```python
from build123d import *

# Parameters (mm, degrees)
SKETCH_W           = 49
SKETCH_H           = 20
PAD_DEPTH          = 2
SKETCH001_W        = 10
SKETCH001_H        = 10
PAD001_DEPTH       = 5
SKETCH002_W        = 13.5
SKETCH002_H        = 10
POCKET_DEPTH       = 5
SKETCH003_W        = 3
SKETCH003_H        = 20
PAD002_DEPTH       = 10
SKETCH004_W        = 1
SKETCH004_H        = 2
PAD003_DEPTH       = 2
PAD003_FACE1_W     = 20
PAD003_FACE1_H     = 2
PAD004_DEPTH       = 2
SKETCH005_W        = 3
SKETCH005_H        = 20
PAD005_DEPTH       = 10
SKETCH006_W        = 1
SKETCH006_H        = 20
PAD006_DEPTH       = 2
PAD006_FACE9_W     = 10
PAD006_FACE9_H     = 2
POCKET001_DEPTH    = 5
SKETCH007_W        = 10
SKETCH007_H        = 2
POCKET002_DEPTH    = 5
POCKET002_FACE22_W = 20
POCKET002_FACE22_H = 1
PAD007_DEPTH       = 5
PAD007_FACE13_W    = 2
PAD007_FACE13_H    = 1
PAD008_DEPTH       = 5
PAD008_FACE22_W    = 2
PAD008_FACE22_H    = 1
PAD009_DEPTH       = 5
PAD009_FACE26_W    = 10
PAD009_FACE26_H    = 10
PAD010_DEPTH       = 15
SKETCH009_W        = 10
SKETCH009_H        = 2
PAD011_DEPTH       = 5
PAD011_FACE29_W    = 10
PAD011_FACE29_H    = 10
PAD012_DEPTH       = 3
SKETCH010_W        = 8
SKETCH010_H        = 2
POCKET003_DEPTH    = 15.001
CHAMFER_SIZE       = 1
CHAMFER_FACE27_W   = 10
CHAMFER_FACE27_H   = 2
PAD013_DEPTH       = 20


with BuildPart() as part:
    # Sketch → Pad (new body)
    with BuildSketch(Plane.XY):
        with Locations((24.5, 10)):
            Rectangle(SKETCH_W, SKETCH_H)
    extrude(amount=PAD_DEPTH)

    # Sketch001 (on Face6 of Pad) → Pad001 (join)
    with BuildSketch(Plane.XY.offset(2)):
        with Locations((24.5, 10)):
            Rectangle(SKETCH001_W, SKETCH001_H)
    extrude(amount=-PAD001_DEPTH)

    # Sketch002 (on Face4 of Pad001) → Pocket (cut)
    with BuildSketch(Plane(origin=(0, 0, 0), x_dir=(1, 0, 0), z_dir=(0, 0, -1))):
        with Locations((39.25, -10)):
            Rectangle(SKETCH002_W, SKETCH002_H)
        with Locations((9.75, -10)):
            Rectangle(SKETCH002_W, SKETCH002_H)
    extrude(amount=-POCKET_DEPTH, mode=Mode.SUBTRACT)

    # Sketch003 (on Face5 of Pocket) → Pad002 (join)
    with BuildSketch(Plane.XY.offset(2)):
        with Locations((47.5, 10)):
            Rectangle(SKETCH003_W, SKETCH003_H)
    extrude(amount=PAD002_DEPTH)

    # Sketch004 (on Face17 of Pad002) → Pad003 (join)
    with BuildSketch(Plane.XY.offset(12)):
        with Locations((48.5, 19)):
            Rectangle(SKETCH004_W, SKETCH004_H)
        with Locations((48.5, 1)):
            Rectangle(SKETCH004_W, SKETCH004_H)
    extrude(amount=PAD003_DEPTH)

    # Pad003 Face1 → Pad004 (add)
    with BuildSketch(Plane(origin=(0, 10, 1), x_dir=(0, 1, 0), z_dir=(-1, 0, 0))):
        Rectangle(PAD003_FACE1_W, PAD003_FACE1_H)
    extrude(amount=PAD004_DEPTH)

    # Sketch005 (on Face26 of Pad004) → Pad005 (join)
    with BuildSketch(Plane.XY.offset(2)):
        with Locations((-0.5, 10)):
            Rectangle(SKETCH005_W, SKETCH005_H)
    extrude(amount=PAD005_DEPTH)

    # Sketch006 (on Face22 of Pad005) → Pad006 (join)
    with BuildSketch(Plane.XY.offset(12)):
        with Locations((-1.5, 10)):
            Rectangle(SKETCH006_W, SKETCH006_H)
    extrude(amount=PAD006_DEPTH)

    # Pad006 Face9 → Pocket001 (cut)
    with BuildSketch(Plane(origin=(3, 10, 1), x_dir=(0, -1, 0), z_dir=(1, 0, 0))):
        Rectangle(PAD006_FACE9_W, PAD006_FACE9_H)
    extrude(amount=-POCKET001_DEPTH, mode=Mode.SUBTRACT)

    # Sketch007 (on Face8 of Pocket001) → Pocket002 (cut)
    with BuildSketch(Plane(origin=(46, 0, 0), x_dir=(0, -1, 0), z_dir=(-1, 0, 0))):
        with Locations((-10, 1)):
            Rectangle(SKETCH007_W, SKETCH007_H)
    extrude(amount=-POCKET002_DEPTH, mode=Mode.SUBTRACT)

    # Pocket002 Face22 → Pad007 (add)
    with BuildSketch(Plane(origin=(-1.5, 10, 14), x_dir=(0, 1, 0), z_dir=(0, 0, 1))):
        Rectangle(POCKET002_FACE22_W, POCKET002_FACE22_H)
    extrude(amount=PAD007_DEPTH)

    # Pad007 Face13 → Pad008 (add)
    with BuildSketch(Plane(origin=(48.5, 1, 14), x_dir=(0, 1, 0), z_dir=(0, 0, 1))):
        Rectangle(PAD007_FACE13_W, PAD007_FACE13_H)
    extrude(amount=PAD008_DEPTH)

    # Pad008 Face22 → Pad009 (add)
    with BuildSketch(Plane(origin=(48.5, 19, 14), x_dir=(0, 1, 0), z_dir=(0, 0, 1))):
        Rectangle(PAD008_FACE22_W, PAD008_FACE22_H)
    extrude(amount=PAD009_DEPTH)

    # Pad009 Face26 → Pad010 (add)
    with BuildSketch(Plane(origin=(24.5, 10, -3), x_dir=(0, -1, 0), z_dir=(0, 0, -1))):
        Rectangle(PAD009_FACE26_W, PAD009_FACE26_H)
    extrude(amount=PAD010_DEPTH)

    # Sketch009 (on Face27 of Pad010) → Pad011 (join)
    with BuildSketch(Plane.XZ.offset(-5)):
        with Locations((24.5, -11)):
            Rectangle(SKETCH009_W, SKETCH009_H)
    extrude(amount=PAD011_DEPTH)

    # Pad011 Face29 → Pad012 (add)
    with BuildSketch(Plane(origin=(24.5, 10, -18), x_dir=(0, -1, 0), z_dir=(0, 0, -1))):
        Rectangle(PAD011_FACE29_W, PAD011_FACE29_H)
    extrude(amount=PAD012_DEPTH)

    # Sketch010 (on Face31 of Pad012) → Pocket003 (cut, through all)
    with BuildSketch(Plane.XZ.offset(-5)):
        with Locations((24.5, -18)):
            Rectangle(SKETCH010_W, SKETCH010_H)
    extrude(amount=-POCKET003_DEPTH, mode=Mode.SUBTRACT)

    # Chamfer
    chamfer_edges = [part.edges().sort_by_distance(p)[0] for p in [
        (24.5, 5, -17),
        (24.5, 5, -19),
        (24.5, 15, -17),
        (24.5, 15, -19),
    ]]
    chamfer(chamfer_edges, length=CHAMFER_SIZE)

    # Chamfer Face27 → Pad013 (add)
    with BuildSketch(Plane(origin=(24.5, 0, -11), x_dir=(-1, 0, 0), z_dir=(0, -1, 0))):
        Rectangle(CHAMFER_FACE27_W, CHAMFER_FACE27_H)
    extrude(amount=-PAD013_DEPTH)


solid = part.part
```
Here's how the part is built. I have some questions about the finished solid (model axes, mm). A direction names the side the tool comes from. Round coordinates to 2 decimals unless told otherwise and drop trailing zeros. Write each loop counter-clockwise with the first axis right and the second up, starting at its lowest first coordinate (ties: lowest second). Pieces come first, ordered by that corner, then holes.
Q1. If we section it at D-D on x = 8: Write out the boundary of the cut face in (y, z), plus the area to 3 significant figures.
Q2. If we section it at B-B on z = 5.5: Write out the boundary of the cut face in (x, y), plus the area to 3 significant figures.
Q3. Will these pins go through, and if not, where does the flat tip stop? P1, Ø10, axis at x = 33.5, y = 5.5, coming from the -Z side; P2, Ø1.5, axis at y = 9.5, z = -0.5, coming from the -X side; P3, Ø5, axis at x = 22.5, z = -4.5, coming from the +Y side; P4, Ø6, axis at x = 40, y = 4.5, coming from the +Z side.
Q4. Please list where these lines run through material, in increasing order: probe 1 along X at (y, z) = (7.75, 4.5); probe 2 along Z at (x, y) = (25.5, 7.25); probe 3 along X at (y, z) = (5.5, -17.5).
Q5. Which directions (+Z, -Z, +X, -X, +Y, -Y) give clear straight access to the entire face, cutting with the end or side of a thin tool? Please do faces 5 (the flat face through (16.5, 10, 1)), 6 (the flat face through (25, 17, -10)), 7 (the flat face through (0, 10, 12)).
Q6. If we section it at A-A on y = 7: Write out the boundary of the cut face in (x, z).
Q7. If we mould it in two halves opening along Y, with no side actions, what happens to faces 1 (the flat face through (7, 15, 1)), 2 (the flat face through (25, 5, -5)), 3 (the flat face through (0, 10, 2)), 4 (the flat face through (30, 10, 0))? For each: +Y half, -Y half, draft (parallel to the pull), parting line (faces both ways), or undercut.
Q8. If we section it at C-C on x = 27.5: Write out the boundary of the cut face in (y, z).
Answer below:
1. outline: (0, 0) - (5, 0) - (5, 2) - (0, 2) - close; (15, 0) - (20, 0) - (20, 2) - (15, 2) - close
1. area: 20.0 mm2
2. outline: (-2, 0) - (1, 0) - (1, 20) - (-2, 20) - close; (46, 0) - (49, 0) - (49, 20) - (46, 20) - close
2. area: 120 mm2
3. P1: stops at z = -21
3. P2: stops at x = 16.5
3. P3: stops at y = 15
3. P4: stops at z = 2
4. probe 1: x = -2 to 1, 46 to 49
4. probe 2: z = -21 to -19, -17 to 2
4. probe 3: x = 19.5 to 20.5, 28.5 to 29.5
5. face 5: +Z, -Z, -X
5. face 6: +X, -X, +Y
5. face 7: +Z, +Y, -Y
6. outline: (-2, 2) - (1, 2) - (1, 12) - (-1, 12) - (-1, 19) - (-2, 19) - close; (16.5, 0) - (19.5, 0) - (19.5, -21) - (29.5, -21) - (29.5, 0) - (32.5, 0) - (32.5, 2) - (16.5, 2) - close; (46, 2) - (49, 2) - (49, 12) - (46, 12) - close; hole (20.5, -19) - (28.5, -19) - (28.5, -17) - (20.5, -17) - close
7. face 1: undercut
7. face 2: -Y half
7. face 3: undercut
7. face 4: draft
8. outline: (0, -12) - (5, -12) - (5, -16) - (6, -17) - (14, -17) - (15, -16) - (15, -12) - (20, -12) - (20, -10) - (15, -10) - (15, 0) - (20, 0) - (20, 2) - (0, 2) - (0, 0) - (5, 0) - (5, -10) - (0, -10) - close; (5, -21) - (15, -21) - (15, -20) - (14, -19) - (6, -19) - (5, -20) - close
